Work out the finished part from the listing and answer in its coordinate system (mm). A direction names the side the tool comes from. Coordinates: 2 decimals unless noted, no trailing zeros. Order: outer loops, then holes, each group sorted by start corner. A loop starts at its lowest first (then second) coordinate and runs counter-clockwise, first axis right, second up. Notation, with made-up numbers: M -19.5,-28 L 5.5,-28 A26 cw 5.5,6 Z; hole C -25,0 d2. An arc over 180 degrees is marked long. Use a Markdown table: item, result. Add a question column.
from build123d import *

# Parameters (mm, degrees)
SKETCH1_W           = 136.525
SKETCH1_H           = 787.4
BOSS_EXTRUDE1_DEPTH = 88.9
SKETCH2_W           = 85.725
SKETCH2_H           = 44.45
BOSS_EXTRUDE2_DEPTH = 25.4
SKETCH4_W           = 44.45
SKETCH4_H           = 495.3
CUT_EXTRUDE1_DEPTH  = 44.45
SKETCH4_3_R         = 31.75
SKETCH4_3_R_2       = 15.875
CUT_EXTRUDE2_DEPTH  = 12.7
SKETCH4_4_R         = 15.875
CUT_EXTRUDE3_DEPTH  = 434.829216289
SKETCH5_W           = 28.575
SKETCH5_H           = 76.2
SKETCH5_W_2         = 15.875
CUT_EXTRUDE4_DEPTH  = 19.05
SKETCH5_3_R         = 4.7625
CUT_EXTRUDE5_DEPTH  = 450.652194062
SKETCH6_W           = 15.875
SKETCH6_H           = 88.9
SKETCH6_H_2         = 69.85
CUT_EXTRUDE6_DEPTH  = 50.8
SKETCH7_R           = 4.7625
CUT_EXTRUDE7_DEPTH  = 44.45
CUT_EXTRUDE8_DEPTH  = 12.7
CUT_EXTRUDE9_DEPTH  = 450.652194062


with BuildPart() as part:
    # Sketch1 → Boss-Extrude1 (new body)
    with BuildSketch(Plane.XY):
        Rectangle(SKETCH1_W, SKETCH1_H)
    extrude(amount=BOSS_EXTRUDE1_DEPTH)

    # Sketch2 → Boss-Extrude2 (add)
    with BuildSketch(Plane(origin=(0, 393.7, 0), x_dir=(1, 0, 0), z_dir=(0, 1, 0))):
        with Locations((0, -50.8)):
            Rectangle(SKETCH2_W, SKETCH2_H)
    extrude(amount=BOSS_EXTRUDE2_DEPTH)

    # Sketch4 → Cut-Extrude1 (cut)
    with BuildSketch(Plane(origin=(0, 0, 0), x_dir=(-1, 0, 0), z_dir=(0, 0, -1))):
        with Locations((0, -120.65)):
            Rectangle(SKETCH4_W, SKETCH4_H)
    extrude(amount=-CUT_EXTRUDE1_DEPTH, mode=Mode.SUBTRACT)

    # Sketch4_3 → Cut-Extrude2 (cut)
    with BuildSketch(Plane(origin=(0, 0, 0), x_dir=(-1, 0, 0), z_dir=(0, 0, -1))):
        with Locations((0, 171.45)):
            Circle(SKETCH4_3_R)
        with Locations((0, 171.45)):
            Circle(SKETCH4_3_R_2, mode=Mode.SUBTRACT)
    extrude(amount=-CUT_EXTRUDE2_DEPTH, mode=Mode.SUBTRACT)

    # Sketch4_4 → Cut-Extrude3 (cut, through all)
    with BuildSketch(Plane(origin=(0, 0, 0), x_dir=(-1, 0, 0), z_dir=(0, 0, -1))):
        with Locations((0, 171.45)):
            Circle(SKETCH4_4_R)
    extrude(amount=-CUT_EXTRUDE3_DEPTH, mode=Mode.SUBTRACT)

    # Sketch5 → Cut-Extrude4 (cut)
    with BuildSketch(Plane.ZY.offset(68.2625)):
        with Locations((30.1625, -212.725)):
            Rectangle(SKETCH5_W, SKETCH5_H)
        with Locations((52.3875, -212.725)):
            Rectangle(SKETCH5_W_2, SKETCH5_H)
    extrude(amount=-CUT_EXTRUDE4_DEPTH, mode=Mode.SUBTRACT)

    # Sketch5_3 → Cut-Extrude5 (cut, through all)
    with BuildSketch(Plane.ZY.offset(68.2625)):
        with Locations(Location((22.225, 104.775, 0), (0, 0, 270))):
            Circle(SKETCH5_3_R)
    extrude(amount=-CUT_EXTRUDE5_DEPTH, mode=Mode.SUBTRACT)

    # Sketch6 → Cut-Extrude6 (cut)
    with BuildSketch(Plane.XY.offset(88.9)):
        with Locations((46.0375, -212.725)):
            Rectangle(SKETCH6_W, SKETCH6_H)
        with Locations((46.0375, 339.725)):
            Rectangle(SKETCH6_W, SKETCH6_H_2)
    extrude(amount=-CUT_EXTRUDE6_DEPTH, mode=Mode.SUBTRACT)

    # Sketch7 → Cut-Extrude7 (cut)
    with BuildSketch(Plane(origin=(68.2625, 0, 0), x_dir=(0, 0, -1), z_dir=(1, 0, 0))):
        with Locations(Location((-63.5, -188.9125, 0), (0, 0, 90))):
            Circle(SKETCH7_R)
        with Locations(Location((-63.5, -236.5375, 0), (0, 0, 90))):
            Circle(SKETCH7_R)
        with Locations(Location((-63.5, 363.5375, 0), (0, 0, 90))):
            Circle(SKETCH7_R)
        with Locations(Location((-63.5, 315.9125, 0), (0, 0, 90))):
            Circle(SKETCH7_R)
    extrude(amount=-CUT_EXTRUDE7_DEPTH, mode=Mode.SUBTRACT)

    # Sketch8 → Cut-Extrude8 (cut)
    with BuildSketch(Plane(origin=(68.2625, 0, 0), x_dir=(0, 0, -1), z_dir=(1, 0, 0))):
        with BuildLine():
            ThreePointArc((-31.75, -212.725), (-25.4, -206.375), (-19.05, -212.725))
            Line((-19.05, -212.725), (-15.875, -212.725))
            Line((-15.875, -212.725), (-15.875, -202.075726257))
            ThreePointArc((-15.875, -202.075726257), (-31.23284745, -199.682356599), (-39.6875, -212.725))
            Line((-39.6875, -212.725), (-31.75, -212.725))
        make_face()
        with BuildLine():
            Line((-15.875, -212.725), (-19.05, -212.725))
            ThreePointArc((-19.05, -212.725), (-25.4, -219.075), (-31.75, -212.725))
            Line((-31.75, -212.725), (-39.6875, -212.725))
            ThreePointArc((-39.6875, -212.725), (-31.23284745, -225.767643401), (-15.875, -223.374273743))
            Line((-15.875, -223.374273743), (-15.875, -212.725))
        make_face()
        with BuildLine():
            Line((-15.875, -202.075726257), (-15.875, -212.725))
            Line((-15.875, -212.725), (-15.875, -223.374273743))
            ThreePointArc((-15.875, -223.374273743), (-12.357356599, -218.55784745), (-11.1125, -212.725))
            ThreePointArc((-11.1125, -212.725), (-12.357356599, -206.89215255), (-15.875, -202.075726257))
        make_face()
    extrude(amount=-CUT_EXTRUDE8_DEPTH, mode=Mode.SUBTRACT)

    # Sketch8_3 → Cut-Extrude9 (cut, through all)
    with BuildSketch(Plane(origin=(68.2625, 0, 0), x_dir=(0, 0, -1), z_dir=(1, 0, 0))):
        with BuildLine():
            ThreePointArc((-31.75, -212.725), (-25.4, -219.075), (-19.05, -212.725))
            Line((-19.05, -212.725), (-31.75, -212.725))
        make_face()
        with BuildLine():
            Line((-31.75, -212.725), (-19.05, -212.725))
            ThreePointArc((-19.05, -212.725), (-25.4, -206.375), (-31.75, -212.725))
        make_face()
    extrude(amount=-CUT_EXTRUDE9_DEPTH, mode=Mode.SUBTRACT)


solid = part.part
(1) The mould has two halves that part along Y. Classify faces 1 (the flat face through (0, -117, 44.45)), 2 (the flat face through (-1, 406, 73.025)): pulls with the +Y half, pulls with the -Y half, needs draft (parallel to the pull), parting line crosses it, or undercut.
(2) A cutting plane is placed at B-B on x = 0. Write down the section's boundary in (y, z) (3 decimals).
(3) Straight lines are drawn through the part: line 1 (X direction, y = -210, z = 43) (1 decimal); line 2 (Y direction, x = 29, z = 63); line 3 (X direction, y = -58, z = 15) (1 decimal). For each, find the intervals that lie inside material, in ascending order.
(4) Which of the six approach directions +Z, -Z, +X, -X, +Y, -Y give full straight-line access (tool end or side, diameter ignored) to faces 3 (the flat face through (-1, 6, 88.9)), 4 (the flat face through (-59, -174.625, 38)), 5 (the cylindrical face through (4.13, 202.93, 6.26)), 6 (the flat face through (68.262, -6, 44)), 7 (the flat face through (46, -168.275, 64))?
(5) Given P1, Ø3, axis at x = -25.5, z = 23, coming from the +Y side; P2, Ø5.5, axis at y = -188.91, z = 63.5, coming from the +X side; P3, Ø16.5, axis at y = -212.725, z = 25.4, coming from the +X side; P4, Ø8.5, axis at y = 104.775, z = 22.225, coming from the +X side (3 decimals), each flat-ended and moving along its own axis, determine where each tip first touches the part or whether it passes through.
(6) A cutting plane is placed at D-D on z = 81. Count the separate pieces of the cut face and the enclosed holes in it, plus the area to 3 significant figures.
From the geometry:
| question | item | result |
|---|---|---|
| 1 | face 1 | undercut |
| 1 | face 2 | needs draft |
| 2 | outline | M -393.7,0 L -368.3,0 L -368.3,44.45 L 127,44.45 L 127,0 L 139.7,0 L 139.7,12.7 L 155.575,12.7 L 155.575,88.9 L -393.7,88.9 Z; M 187.325,12.7 L 203.2,12.7 L 203.2,0 L 393.7,0 L 393.7,28.575 L 419.1,28.575 L 419.1,73.025 L 393.7,73.025 L 393.7,88.9 L 187.325,88.9 Z |
| 3 | line 1 | x = -49.2 to -22.2, 22.2 to 38.1, 54 to 68.3 |
| 3 | line 2 | y = -393.7 to -241.27, -231.8 to -193.65, -184.18 to 311.18, 320.65 to 358.8, 368.27 to 419.1 |
| 3 | line 3 | x = -68.3 to -22.2, 22.2 to 68.3 |
| 4 | face 3 | +Z, +X, -X, +Y, -Y |
| 4 | face 4 | -X |
| 4 | face 5 | -Z |
| 4 | face 6 | +Z, -Z, +X, +Y, -Y |
| 4 | face 7 | +Z |
| 5 | P1 | stops at y = 393.7 |
| 5 | P2 | stops at x = 23.81 |
| 5 | P3 | stops at x = 55.56 |
| 5 | P4 | passes through |
| 6 | separate pieces | 1 |
| 6 | enclosed holes | 3 |
| 6 | area | 104,000 mm2 |
